```python
from build123d import *

# Parameters (mm, degrees)
SKIZZE1_W                       = 16
SKIZZE1_H                       = 16
SKIZZE1_W_2                     = 14
SKIZZE1_H_2                     = 14
AUFSATZ_LINEAR_AUSTRAGEN1_DEPTH = 15
SKIZZE2_R                       = 2.5
SCHNITT_LINEAR_AUSTRAGEN1_DEPTH = 30
SKIZZE3_R                       = 5
SCHNITT_LINEAR_AUSTRAGEN2_DEPTH = 5


with BuildPart() as part:
    # Skizze1 → Aufsatz-Linear austragen1 (new, symmetric)
    with BuildSketch(Plane.XY):
        Rectangle(SKIZZE1_W, SKIZZE1_H)
        Rectangle(SKIZZE1_W_2, SKIZZE1_H_2, mode=Mode.SUBTRACT)
    extrude(amount=AUFSATZ_LINEAR_AUSTRAGEN1_DEPTH, both=True)

    # Skizze2 → Schnitt-Linear austragen1 (cut)
    with BuildSketch(Plane(origin=(0, 8, 0), x_dir=(1, 0, 0), z_dir=(0, 1, 0))):
        with Locations(Location((0, 0, 0), (0, 0, 270))):
            Circle(SKIZZE2_R)
    extrude(amount=-SCHNITT_LINEAR_AUSTRAGEN1_DEPTH, mode=Mode.SUBTRACT)

    # Skizze3 → Schnitt-Linear austragen2 (cut)
    with BuildSketch(Plane(origin=(0, 8, 0), x_dir=(1, 0, 0), z_dir=(0, 1, 0))):
        with Locations(Location((0, 0, 0), (0, 0, 270))):
            Circle(SKIZZE3_R)
    extrude(amount=-SCHNITT_LINEAR_AUSTRAGEN2_DEPTH, mode=Mode.SUBTRACT)


solid = part.part
```
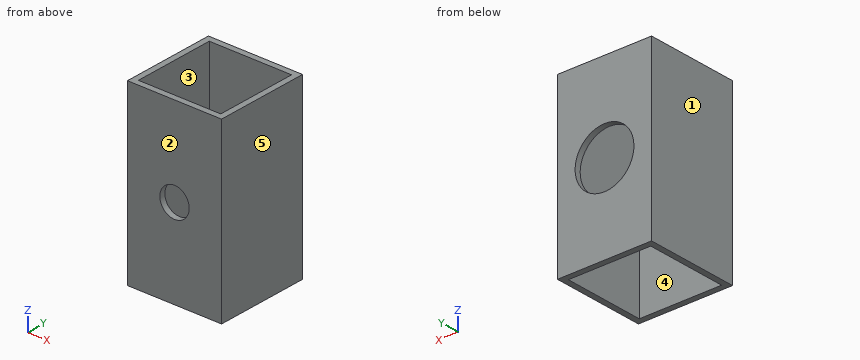
Check sheet for the modelled part. Datum: model origin and axes. Units: mm. Face numbers are marked on the shaded views. A direction names the side the tool comes from. Round coordinates to 2 decimals unless told otherwise and drop trailing zeros. Loops run counter-clockwise (first coordinate to the right, second up) from the corner with the lowest first, then second, coordinate; pieces in that order, holes last. Notation, with made-up numbers: (60.5, 8) -> (99.5, 8) arc R22 ccw to (99.5, 34) -> close; hole circle Ø10 at (-29, 13.5). An arc over 180 degrees is marked (long way). Answer in a Markdown table with one row per item.
Q1. Release check for a two-part mould opening along Y. For the marked faces 1, 2 and 3 record: released by +Y, released by -Y, zero draft, split by the parting line, or undercut.
Data:
| item | result |
|---|---|
| face 1 | zero draft |
| face 2 | released by -Y |
| face 3 | undercut |
Q2. Go/stop test with a flat-tipped pin: P1, Ø6.5, axis at x = 0, z = 0, coming from the +Y side. Record where the tip stops, or that it passes through.
Data:
| item | result |
|---|---|
| P1 | stops at y = -7 |
Q3. Sectioned sample at B-B on z = 0. Enter the section's corners in (x, y).
Data:
| item | result |
|---|---|
| outline | (-8, -8) -> (-2.5, -8) -> (-2.5, -7) -> (-7, -7) -> (-7, 7) -> (-5, 7) -> (-5, 8) -> (-8, 8) -> close; (2.5, -8) -> (8, -8) -> (8, 8) -> (5, 8) -> (5, 7) -> (7, 7) -> (7, -7) -> (2.5, -7) -> close |
Q4. Set-up check for the marked faces 4 and 5: record each of +Z, -Z, +X, -X, +Y, -Y from which the full face is reachable in a straight line by a thin tool's end or side.
Data:
| item | result |
|---|---|
| face 4 | +Z, -Z |
| face 5 | +Z, -Z, +X, +Y, -Y |
Q5. Sectioned sample at C-C on z = -11.5. Enter the section's corners in (x, y), then the cut area to 3 significant figures.
Data:
| item | result |
|---|---|
| outline | (-8, -8) -> (8, -8) -> (8, 8) -> (-8, 8) -> close; hole (-7, -7) -> (7, -7) -> (7, 7) -> (-7, 7) -> close |
| area | 60.0 mm^2 |
Q6. Sectioned sample at A-A on x = -5.5. Enter the section's corners in (y, z).
Data:
| item | result |
|---|---|
| outline | (-8, -15) -> (-7, -15) -> (-7, 15) -> (-8, 15) -> close; (7, -15) -> (8, -15) -> (8, 15) -> (7, 15) -> close |
Q7. Thickness scan on L1, parallel to X at y = 6, z = 11.5; L2, parallel to X at y = 7.75, z = 0. Record the ranges inside material, lowest first.
Data:
| item | result |
|---|---|
| L1 | x = -8 to -7, 7 to 8 |
| L2 | x = -8 to -5, 5 to 8 |
